from build123d import *

# Parameters (mm, degrees)
BOX031_W     = 54
BOX031_H     = 14
BOX031_DEPTH = 15
BOX022_W     = 54
BOX022_H     = 16
BOX022_DEPTH = 17
FILLET_R     = 6.9
FILLET001_R  = 6.9


with BuildPart() as obj1:
    # Box031 → Box031 (new body)
    with BuildSketch(Plane(origin=(-9, 0, -21), x_dir=(1, 0, 0), z_dir=(0, 0, 1))):
        with Locations((27, 7)):
            Rectangle(BOX031_W, BOX031_H)
    extrude(amount=BOX031_DEPTH)


with BuildPart() as fillet001:
    # Box022 → Box022 (new body)
    with BuildSketch(Plane(origin=(-10, -1, -22), x_dir=(1, 0, 0), z_dir=(0, 0, 1))):
        with Locations((27, 8)):
            Rectangle(BOX022_W, BOX022_H)
    extrude(amount=BOX022_DEPTH)

    # Cut: cut obj1
    add(obj1.part, mode=Mode.SUBTRACT)

    # Fillet
    fillet_edges = [fillet001.edges().sort_by_distance(p)[0] for p in [
        (17.5, 0, -21),
    ]]
    fillet(fillet_edges, radius=FILLET_R)

    # Fillet001
    fillet001_edges = [fillet001.edges().sort_by_distance(p)[0] for p in [
        (17.5, 14, -21),
    ]]
    fillet(fillet001_edges, radius=FILLET001_R)


solid = fillet001.part
Input: part model. Units: mm. Frame: model coordinates. A direction names the side the tool comes from. Round coordinates to 2 decimals unless told otherwise and drop trailing zeros. Order: outer loops, then holes, each group sorted by start corner. A loop starts at its lowest first (then second) coordinate and runs counter-clockwise, first axis right, second up. Notation, with made-up numbers: (-34.75, 50) - (-20.75, 50) arc R17 cw to (-20.75, 74) - close; hole circle Ø4 at (19, -2.5). An arc over 180 degrees is marked (long way). Answer as a JSON object with one key per item and string values. Group by question number.
(1) Cut plane B-B (z = -9.75). Return loops of the section in (x, y).
(2) Reachability of faces 1 (the face through (44, 1, -18)), 2 (the face through (-9, 7, -14)) from +Z, -Z, +X, -X, +Y, -Y: full face, straight path, thin tool, end or side. Return the list, or none.
(3) Cut plane A-A (x = 11). Return loops of the section in (y, z), then the cut area to 3 significant figures.
(4) Draft query along Z for faces 3 (the face through (17, 7, -22)), 4 (the face through (17, 0, -10)), 5 (the face through (17, 7, -5)). Return one class per face: released by +Z, released by -Z, zero draft, split by the parting line, or undercut.
(5) Cut plane C-C (y = 12.25). Return loops of the section in (x, z), then the cut area to 3 significant figures.
(6) Material intervals for probe 1 along Z at (x, y) = (32, 7.5); probe 2 along Y at (x, z) = (-4, -10); probe 3 along X at (y, z) = (9, -19.75), sorted ascending. Write a range as from..to.
Here are the results:
{
 "1": {"outline": "(-10, -1) - (44, -1) - (44, 0) - (-9, 0) - (-9, 14) - (44, 14) - (44, 15) - (-10, 15) - close"},
 "2": {"face 1": "+Z, -Z, +X, +Y, -Y", "face 2": "+X"},
 "3": {"outline": "(-1, -22) - (15, -22) - (15, -5) - (-1, -5) - close; hole (0, -14.1) arc R6.9 ccw to (6.9, -21) - (7.1, -21) arc R6.9 ccw to (14, -14.1) - (14, -6) - (0, -6) - close", "area": "82.4 mm^2"},
 "4": {"face 3": "released by -Z", "face 4": "undercut", "face 5": "released by +Z"},
 "5": {"outline": "(-10, -22) - (44, -22) - (44, -18.69) - (-9, -18.69) - (-9, -6) - (44, -6) - (44, -5) - (-10, -5) - close", "area": "245 mm^2"},
 "6": {"probe 1": "z = -22..-20.99, -6..-5", "probe 2": "y = -1..0, 14..15", "probe 3": "x = -10..-9"}
}
